Autodesk Inventor part; units mm, degrees
ref_plane "YZ Plane" through (0, 0, 0) normal (1, 0, 0) x (0, 1, 0)
ref_plane "XZ Plane" through (0, 0, 0) normal (0, 1, 0) x (-1, 0, 0)
ref_plane "XY Plane" through (0, 0, 0) normal (0, 0, 1) x (1, 0, 0)
sketch "Sketch1" plane through (0, 0, 0) normal (1, 0, 0) x (0, 1, 0)
  circle A0 centre (0, 0) radius 3.1
  arc A1 (0, 5) -> (0, -5) centre (0, 0) ccw
  line L0 (0, 5) -> (50, 5)
  line L1 (50, -5) -> (0, -5)
  arc A2 (50, -5) -> (50, 5) centre (50, 0) ccw
  circle A3 centre (50, 0) radius 3.1
  dimension "d0" = 6.2
  dimension "d1" = 10
  dimension "d3" = 50
  dimension "d5" = 6.2
  dimension "d26" = 5
extrude "Extrusion1" add sketch "Sketch1" along normal blind 3
ref_plane "Work Plane1" through (-2, 0, 0) normal (1, 0, 0) x (0, 0, -1)
sketch "Sketch5" plane through (3, 0, 0) normal (1, 0, 0) x (0, 0, -1)
  line L0 (-5, 50) -> (-5, 0)
  arc A0 (-5, 0) -> (5, 0) centre (0, 0) ccw
  circle A1 centre (0, 50) radius 3.1
  circle A2 centre (0, 0) radius 3.1
  arc A3 (-5, 0) -> (5, 0) centre (0, 0) ccw
  line L1 (5, 0) -> (5, 50)
  arc A4 (5, 50) -> (-5, 50) centre (0, 50) ccw
  line L2 (-5, 50) -> (-5, 0)
  line L3 (0, -5) -> (0, 6)
  line L4 (0, 6) -> (5, 11)
  line L5 (5, 0) -> (5, 50)
  line L6 (0, 6) -> (-5, 11)
  line L7 (0, 55) -> (0, 44)
  line L8 (0, 44) -> (-5, 39)
  line L9 (0, 44) -> (5, 39)
  line L10 (0, 44) -> (7.0711, 44) construction
  dimension "d27" = 11
  dimension "d28" = 135
  dimension "d29" = 11
  dimension "d30" = 135
  dimension "d31" = 45
extrude "Extrusion5" cut sketch "Sketch5" against normal blind 10 contours A4 L7 A1 L8 L0 | A4 L1 L9 L7 A1 | L6 L3 A2 A0 L0 | L7 A1 | A1 L7 | L4 L1 A0 L3 A2 | L3 A2 | A2 L3
equation "\"d5\" = d0"
equation "\"d26\" = 0.5 * d1"
equation "\"d29\" = d27"
equation "\"d30\" = d28"
properties part number "ArmSpanMid_01"
Here's how the part is built. I have some questions about the finished solid (model axes, mm). Round coordinates to 2 decimals unless told otherwise and drop trailing zeros. Write each loop counter-clockwise with the first axis right and the second up, starting at its lowest first coordinate (ties: lowest second). Pieces come first, ordered by that corner, then holes.
1. Suppose I cut it at B-B (z = 4.25). List the corners of the cut face in (x, y) for me.
2. Suppose I cut it at A-A (x = 0.8). List the corners of the cut face in (y, z) for me, and give its area (3 significant figures).
3. I need wall thicknesses on L1, parallel to Y at x = 1.8, z = -2; L2, parallel to Y at x = 1.8, z = 4; L3, parallel to Z at x = 1.5, y = 10. Which ranges of each line are inside material? Lowest first, please.
4. Will this pin go through, and if not, where does the flat tip stop? pin 1 Ø4 at (y, z) = (31, 3) entering from -X.
5. Suppose I cut it at C-C (z = -1.75). List the corners of the cut face in (x, y) for me.
Answer sheet:
1. outline: (0, 10.25) - (3, 10.25) - (3, 39.75) - (0, 39.75) - close
2. outline: (6, 0) - (11, -5) - (39, -5) - (44, 0) - (39, 5) - (11, 5) - close
2. area: 330 mm2
3. L1: y = 8 to 42
3. L2: y = 10 to 40
3. L3: z = -4 to 4
4. pin 1: stops at x = 0
5. outline: (0, 7.75) - (3, 7.75) - (3, 42.25) - (0, 42.25) - close
